Verification items for the finished model (mm, model axes). Face numbers are marked on the shaded views. A direction names the side the tool comes from. Round coordinates to 2 decimals unless told otherwise and drop trailing zeros. Order: outer loops, then holes, each group sorted by start corner. A loop starts at its lowest first (then second) coordinate and runs counter-clockwise, first axis right, second up. Notation, with made-up numbers: (83, -26.5) -> (94, -26.5) arc R26 cw to (94, -7.5) -> close; hole circle Ø1 at (38.5, 57.5). An arc over 180 degrees is marked (long way). Put each result on its own line as item: value.
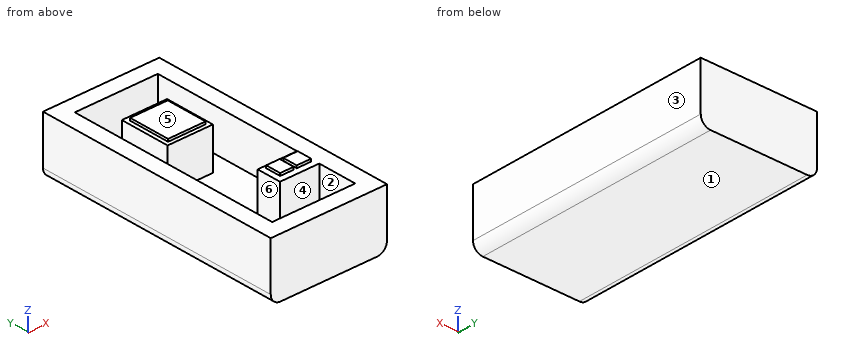
from build123d import *

# Parameters (mm, degrees)
F0_W     = 177.8
F0_H     = 88.9
F1_DEPTH = 381
F2_T     = -25.4
F3_W     = 69.2884027958
F3_H     = 76.5359997749
F3_W_2   = 60.1096697411
F3_H_2   = 37.3346805573
F4_DEPTH = 63.5
F5_W     = 57.4366301298
F5_H     = 63.3930116892
F5_W_2   = 22.1205726266
F5_H_2   = 22.5539207458
F5_W_3   = 20.6655599177
F5_H_3   = 23.4381556511
F6_DEPTH = 3.81
F7_R     = 15
F8_R     = 15


with BuildPart() as f1:
    # F0 (on Front) → F1 (new body)
    with BuildSketch(Plane.XZ):
        with Locations((1.1990362685, 0)):
            Rectangle(F0_W, F0_H)
    extrude(amount=F1_DEPTH)

    # F2
    f2_openings = [f1.faces().sort_by_distance(p)[0] for p in [
        (1.199036, -190.5, 44.45),
    ]]
    offset(amount=F2_T, openings=f2_openings)

    # F3 (on face) → F4 (join)
    with BuildSketch(Plane.XY.offset(-19.05)):
        with Locations((0, -112.0956093073)):
            Rectangle(F3_W, F3_H)
        with Locations((34.6442013979, -276.8346965313)):
            Rectangle(F3_W_2, F3_H_2)
    extrude(amount=F4_DEPTH)

    # F5 (on face) → F6 (join)
    with BuildSketch(Plane.XY.offset(44.45)):
        with Locations((0, -112.9631772637)):
            Rectangle(F5_W, F5_H)
        with Locations((49.8413220048, -274.8637795448)):
            Rectangle(F5_W_2, F5_H_2)
        with Locations((23.7438436598, -274.4216620922)):
            Rectangle(F5_W_3, F5_H_3)
    extrude(amount=F6_DEPTH)

    # F7
    f7_edges = [f1.edges().sort_by_distance(p)[0] for p in [
        (90.099036, -190.5, -44.45),
    ]]
    fillet(f7_edges, radius=F7_R)

    # F8
    f8_edges = [f1.edges().sort_by_distance(p)[0] for p in [
        (-87.700964, -190.5, -44.45),
    ]]
    fillet(f8_edges, radius=F8_R)


solid = f1.part
Item 1: Material ranges on L1, parallel to Y at x = -33.5, z = -18.5; L2, parallel to X at y = -130.5, z = 29.5; L3, parallel to X at y = -233.5, z = 28, recorded low to high. Write a range as [from, to].
Check sheet entries:
L1: y = [-381, -355.6], [-150.36, -73.83], [-25.4, 0]
L2: x = [-87.7, -62.3], [-34.64, 34.64], [64.7, 90.1]
L3: x = [-87.7, -62.3], [64.7, 90.1]
Item 2: Tool access check on the marked faces 5 and 6. Record the directions out of +Z, -Z, +X, -X, +Y, -Y that give a thin tool (end or side, any length) a straight path to the whole face; none if there is none.
Check sheet entries:
face 5: +Z, +X, -X, +Y, -Y
face 6: +Z
Item 3: Gauge pin test, flat ends, axial feed: pin 1 Ø18 at (x, z) = (48, 25.5) entering from +Y; pin 2 Ø3 at (x, z) = (52, 47) entering from -Y; pin 3 Ø1.1 at (x, z) = (50.5, 46) entering from +Y; pin 4 Ø1.9 at (y, z) = (-275.5, 47) entering from +X. Record the tip position at first contact, or that the pin passes through.
Check sheet entries:
pin 1: stops at y = 0
pin 2: stops at y = -286.14
pin 3: stops at y = -263.59
pin 4: stops at x = 60.9
Item 4: Section check B-B on y = -33. Record the boundary of the cut face in (x, z).
Check sheet entries:
outline: (-87.7, -29.45) arc R15 ccw to (-72.7, -44.45) -> (75.1, -44.45) arc R15 ccw to (90.1, -29.45) -> (90.1, 44.45) -> (64.7, 44.45) -> (64.7, -19.05) -> (-62.3, -19.05) -> (-62.3, 44.45) -> (-87.7, 44.45) -> close
Item 5: Section check D-D on x = -23. Record the boundary of the cut face in (y, z).
Check sheet entries:
outline: (-381, -44.45) -> (0, -44.45) -> (0, 44.45) -> (-25.4, 44.45) -> (-25.4, -19.05) -> (-73.83, -19.05) -> (-73.83, 44.45) -> (-81.27, 44.45) -> (-81.27, 48.26) -> (-144.66, 48.26) -> (-144.66, 44.45) -> (-150.36, 44.45) -> (-150.36, -19.05) -> (-355.6, -19.05) -> (-355.6, 44.45) -> (-381, 44.45) -> close
Item 6: Section check C-C on x = 9. Record the boundary of the cut face in (y, z).
Check sheet entries:
outline: (-381, -44.45) -> (0, -44.45) -> (0, 44.45) -> (-25.4, 44.45) -> (-25.4, -19.05) -> (-73.83, -19.05) -> (-73.83, 44.45) -> (-81.27, 44.45) -> (-81.27, 48.26) -> (-144.66, 48.26) -> (-144.66, 44.45) -> (-150.36, 44.45) -> (-150.36, -19.05) -> (-258.17, -19.05) -> (-258.17, 44.45) -> (-295.5, 44.45) -> (-295.5, -19.05) -> (-355.6, -19.05) -> (-355.6, 44.45) -> (-381, 44.45) -> close
Item 7: Section check A-A on z = -7.5. Record the boundary of the cut face in (x, y), then the cut area to 3 significant figures.
Check sheet entries:
outline: (-87.7, -381) -> (90.1, -381) -> (90.1, 0) -> (-87.7, 0) -> close; (-34.64, -150.36) -> (34.64, -150.36) -> (34.64, -73.83) -> (-34.64, -73.83) -> close; hole (-62.3, -355.6) -> (64.7, -355.6) -> (64.7, -295.5) -> (4.59, -295.5) -> (4.59, -258.17) -> (64.7, -258.17) -> (64.7, -25.4) -> (-62.3, -25.4) -> close
area: 33,400 mm^2
Item 8: Release check for a two-part mould opening along X. For the marked faces 1, 2, 3 and 4 record: +X half, -X half, draft (parallel to the pull), parting line (faces both ways), or undercut.
Check sheet entries:
face 1: draft
face 2: undercut
face 3: +X half
face 4: undercut
